Design review of the part built by this model. Coordinates are the model's own, in mm. Coordinates: 2 decimals unless noted, no trailing zeros. Order: outer loops, then holes, each group sorted by start corner. A loop starts at its lowest first (then second) coordinate and runs counter-clockwise, first axis right, second up. Notation, with made-up numbers: M -8,-37.5 L 30,-37.5 A30 ccw 30,-10.5 Z; hole C 88.25,31.5 d1. An arc over 180 degrees is marked long. Use CSV: the item, a comma, the result in double quotes.
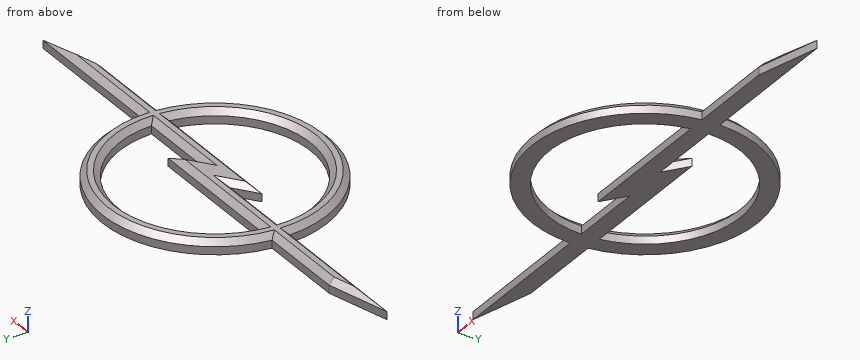
```python
from build123d import *

# Parameters (mm, degrees)
F1_DEPTH = 3.048
F2_SIZE  = 1.27


with BuildPart() as f1:
    # F0 (on Top) → F1 (new body)
    with BuildSketch(Plane.XY):
        with BuildLine():
            Line((-25.112624, 3.81), (-44.45, 3.81))
            Line((-44.45, 3.81), (-58.42, 0))
            Line((-58.42, 0), (-25.4, 0))
            ThreePointArc((-25.4, 0), (-1.910411, -25.328054), (25.112624, -3.81))
            Line((25.112624, -3.81), (44.45, -3.81))
            Line((44.45, -3.81), (58.42, 0))
            Line((58.42, 0), (25.4, 0))
            ThreePointArc((25.4, 0), (1.910411, 25.328054), (-25.112624, 3.81))
        make_face()
        with BuildLine():
            Line((-5.08, 0), (-10.16, -3.81))
            Line((-10.16, -3.81), (21.251165, -3.81))
            ThreePointArc((21.251165, -3.81), (-1.912519, -21.505124), (-21.59, 0))
            Line((-21.59, 0), (-5.08, 0))
        make_face(mode=Mode.SUBTRACT)
        with BuildLine():
            Line((5.08, 0), (10.16, 3.81))
            Line((10.16, 3.81), (-21.251165, 3.81))
            ThreePointArc((-21.251165, 3.81), (1.912519, 21.505124), (21.59, 0))
            Line((21.59, 0), (5.08, 0))
        make_face(mode=Mode.SUBTRACT)
    extrude(amount=F1_DEPTH)

    # F2
    f2_edges = [f1.edges().sort_by_distance(p)[0] for p in [
        (-51.435, 1.905, 3.048),
        (-34.781312, 3.81, 3.048),
        (-41.91, 0, 3.048),
        (-1.910411, -25.328054, 3.048),
        (-1.912519, -21.505124, 3.048),
        (5.545582, -3.81, 3.048),
        (13.335, 0, 3.048),
        (7.62, 1.905, 3.048),
        (-5.545582, 3.81, 3.048),
        (-13.335, 0, 3.048),
        (-7.62, -1.905, 3.048),
        (1.912519, 21.505124, 3.048),
        (1.910411, 25.328054, 3.048),
        (41.91, 0, 3.048),
        (34.781312, -3.81, 3.048),
        (51.435, -1.905, 3.048),
    ]]
    chamfer(f2_edges, length=F2_SIZE)


solid = f1.part
```
(1) Wall thickness on probe 1 along Y at (x, z) = (2.5, 1.05); probe 2 along Y at (x, z) = (-11, 1.1); probe 3 along Y at (x, z) = (8, 2.2): over which ranges is each line inside the solid? List them lowest first.
The answers:
probe 1,"y = -25.28 to -21.44, -3.81 to 3.81, 21.44 to 25.28"
probe 2,"y = -22.89 to -18.58, 0 to 3.81, 18.58 to 22.89"
probe 3,"y = -23.66 to -20.51, -3.39 to -0.42, 2.72 to 3.39, 20.51 to 23.66"
(2) Add section C-C on x = 33. State the section outline as (y, z) points, and give its area (4 significant figures).
The answers:
outline,"M -3.81,0 L 0,0 L 0,1.78 L -1.27,3.05 L -2.54,3.05 L -3.81,1.78 Z"
area,"10.00 mm2"
(3) Add section A-A on z = 0.9. State the section outline as (x, y) points.
The answers:
outline,"M -58.42,0 L -25.4,0 A25.4 ccw 25.11,-3.81 L 44.45,-3.81 L 58.42,0 L 25.4,0 A25.4 ccw -25.11,3.81 L -44.45,3.81 Z; hole M -21.59,0 A21.59 ccw 21.25,-3.81 L -10.16,-3.81 L -5.08,0 Z; hole M -21.25,3.81 L 10.16,3.81 L 5.08,0 L 21.59,0 A21.59 ccw Z"
(4) Clearance check with flat-ended pins moving along their axes: P1, Ø1.4, axis at x = -38, z = 1, coming from the +Y side; P2, Ø1.4, axis at x = 36, z = 1, coming from the -Y side; P3, Ø1.4, axis at x = -49.5, z = 1, coming from the -Y side. State where each tip first meets the part, or that it passes through.
The answers:
P1,"stops at y = 3.81"
P2,"stops at y = -3.81"
P3,"stops at y = 0"
(5) Add section B-B on x = 0. State the section outline as (y, z) points, and give its area (3 significant figures).
The answers:
outline,"M -25.4,0 L -21.59,0 L -21.59,1.78 L -22.86,3.05 L -24.13,3.05 L -25.4,1.78 Z; M -3.81,0 L 3.81,0 L 3.81,1.78 L 2.54,3.05 L -2.54,3.05 L -3.81,1.78 Z; M 21.59,0 L 25.4,0 L 25.4,1.78 L 24.13,3.05 L 22.86,3.05 L 21.59,1.78 Z"
area,"41.6 mm2"
